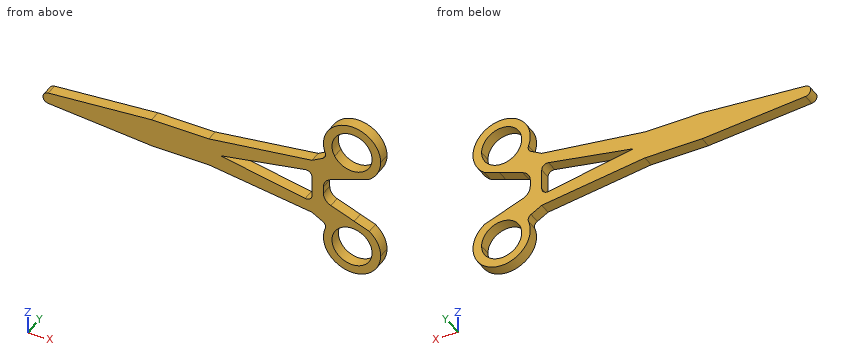
```python
from build123d import *

# Parameters (mm, degrees)
F1_DEPTH = 2
F2_R     = 2
F3_R     = 1


with BuildPart() as f1:
    # F0 (on Front) → F1 (new body)
    with BuildSketch(Plane.XZ):
        with BuildLine():
            Line((30, 2.5), (0, 0))
            Line((0, 0), (42, 0))
            Line((42, 0), (58, 3))
            Line((58, 3), (58, 0))
            Line((58, 0), (60, 0))
            Line((60, 0), (60, 2))
            Line((60, 2), (65.3698630137, 4.0136986301))
            ThreePointArc((65.3698630137, 4.0136986301), (62.6521442193, 4.5855268454), (60.6587842894, 6.5193053082))
            Line((60.6587842894, 6.5193053082), (58, 5))
            Line((58, 5), (40, 2.5))
            Line((40, 2.5), (30, 2.5))
        make_face()
        with BuildLine():
            Line((42, 0), (0, 0))
            Line((0, 0), (30, -2.5))
            Line((30, -2.5), (40, -2.5))
            Line((40, -2.5), (58, -5))
            Line((58, -5), (60.6587842894, -6.5193053082))
            ThreePointArc((60.6587842894, -6.5193053082), (62.6521442193, -4.5855268454), (65.3698630137, -4.0136986301))
            Line((65.3698630137, -4.0136986301), (60, -2))
            Line((60, -2), (60, 0))
            Line((60, 0), (58, 0))
            Line((58, 0), (58, -3))
            Line((58, -3), (42, 0))
        make_face()
        with BuildLine():
            ThreePointArc((70, 9), (63.7166603242, 13.8324982438), (60.6587842894, 6.5193053082))
            ThreePointArc((60.6587842894, 6.5193053082), (62.6521442193, 4.5855268454), (65.3698630137, 4.0136986301))
            Line((65.3698630137, 4.0136986301), (68, 5))
            ThreePointArc((68, 5), (69.472135955, 6.7639320225), (70, 9))
        make_face()
        with BuildLine():
            ThreePointArc((68.5, 9), (65.898337773, 5.6172512293), (61.9611490026, 7.2635137158))
            ThreePointArc((61.9611490026, 7.2635137158), (64.101662227, 12.3827487707), (68.5, 9))
        make_face(mode=Mode.SUBTRACT)
        with BuildLine():
            ThreePointArc((65.3698630137, -4.0136986301), (62.6521442193, -4.5855268454), (60.6587842894, -6.5193053082))
            ThreePointArc((60.6587842894, -6.5193053082), (63.7166603242, -13.8324982438), (70, -9))
            ThreePointArc((70, -9), (69.472135955, -6.7639320225), (68, -5))
            Line((68, -5), (65.3698630137, -4.0136986301))
        make_face()
        with BuildLine():
            ThreePointArc((68.5, -9), (64.101662227, -12.3827487707), (61.9611490026, -7.2635137158))
            ThreePointArc((61.9611490026, -7.2635137158), (65.898337773, -5.6172512293), (68.5, -9))
        make_face(mode=Mode.SUBTRACT)
    extrude(amount=F1_DEPTH)

    # F2
    f2_edges = [f1.edges().sort_by_distance(p)[0] for p in [
        (60, -1, 2),
        (60, -1, -2),
    ]]
    fillet(f2_edges, radius=F2_R)

    # F3
    f3_edges = [f1.edges().sort_by_distance(p)[0] for p in [
        (58, -1, 3),
        (58, -1, -3),
        (60.658784, -1, -6.519305),
        (60.658784, -1, 6.519305),
        (0, -1, 0),
    ]]
    fillet(f3_edges, radius=F3_R)


solid = f1.part
```
Here's how the part is built. I have some questions about the finished solid (model axes, mm). Coordinates: 2 decimals unless noted, no trailing zeros. Loops run counter-clockwise (first coordinate to the right, second up) from the corner with the lowest first, then second, coordinate; pieces in that order, holes last. Notation, with made-up numbers: (70.25, 61) - (122.25, 61) arc R17 cw to (122.25, 82) - close; hole circle Ø5 at (50, -27.5). An arc over 180 degrees is marked (long way). Return JSON: item names as keys, results as strings. Group by question number.
Item 1: If we section it at B-B on x = 17.5: Write out the boundary of the cut face in (y, z).
Item 2: If we section it at C-C on x = 25: Write out the boundary of the cut face in (y, z), and give its area (3 significant figures).
Item 3: If we section it at A-A on y = -0.3: Write out the boundary of the cut face in (x, z).
Item 4: I need wall thicknesses on line 1 (X direction, y = -0.6, z = -9); line 2 (Z direction, x = 65, y = -0.4) (3 decimals); line 3 (Z direction, x = 46, y = -1.1). Which ranges of each line are inside material? Lowest first, please. Write a range as from..to.
Item 5: Will these pins go through, and if not, where does the flat tip stop? P1, Ø8, axis at x = 40.5, z = 10.5, coming from the -Y side; P2, Ø1, axis at x = 34.5, y = -1, coming from the +Z side; P3, Ø1, axis at y = -0.5, z = 0, coming from the +X side.
Calculated:
{
 "1": {"outline": "(-2, -1.46) - (0, -1.46) - (0, 1.46) - (-2, 1.46) - close"},
 "2": {"outline": "(-2, -2.08) - (0, -2.08) - (0, 2.08) - (-2, 2.08) - close", "area": "8.33 mm^2"},
 "3": {"outline": "(11.96, -1) - (30, -2.5) - (40, -2.5) - (58, -5) - (59.86, -6.06) arc R1 cw to (60.31, -7.28) arc R5 ccw (long way) to (68, -5) - (61.3, -2.49) arc R2 cw to (60, -0.61) - (60, 0.61) arc R2 cw to (61.3, 2.49) - (68, 5) arc R5 ccw (long way) to (60.31, 7.28) arc R1 cw to (59.86, 6.06) - (58, 5) - (40, 2.5) - (30, 2.5) - (11.96, 1) arc R1 ccw to start; hole (42, 0) - (56.82, -2.78) arc R1 ccw to (58, -1.8) - (58, 1.8) arc R1 ccw to (56.82, 2.78) - close; hole circle Ø7 at (65, -9); hole circle Ø7 at (65, 9)"},
 "4": {"line 1": "x = 60..61.5, 68.5..70", "line 2": "z = -14..-12.5, -5.5..-3.875, 3.875..5.5, 12.5..14", "line 3": "z = -3.33..-0.75, 0.75..3.33"},
 "5": {"P1": "passes through", "P2": "stops at z = 2.5", "P3": "stops at x = 60"}
}
